Design review of the part built by this model. Coordinates are the model's own, in mm. Face numbers are marked on the shaded views. A direction names the side the tool comes from. Round coordinates to 2 decimals unless told otherwise and drop trailing zeros. Order: outer loops, then holes, each group sorted by start corner. A loop starts at its lowest first (then second) coordinate and runs counter-clockwise, first axis right, second up.
from build123d import *

# Parameters (mm, degrees)
F1_DEPTH = 25.4
F2_R     = 30.191545
F2_R_2   = 13.204956
F3_DEPTH = 46.73447
F4_W     = 33.58691
F4_H     = 33.58691
F5_DEPTH = 38.1


with BuildPart() as f1:
    # F0 (on Right) → F1 (new body)
    with BuildSketch(Plane.YZ):
        with BuildLine():
            ThreePointArc((-64.193385, -51.494292), (-34.284922, -33.102834), (-22.581748, 0))
            ThreePointArc((-22.581748, 0), (-34.284922, 33.102834), (-64.193385, 51.494292))
            ThreePointArc((-64.193385, 51.494292), (-127.917436, 0), (-64.193385, -51.494292))
        make_face()
        with BuildLine():
            ThreePointArc((-64.193385, 51.494292), (-34.284922, 33.102834), (-22.581748, 0))
            ThreePointArc((-22.581748, 0), (-34.284922, -33.102834), (-64.193385, -51.494292))
            Line((-64.193385, -51.494292), (59.976784, -24.834034))
            ThreePointArc((59.976784, -24.834034), (29.244732, 0), (59.976784, 24.834034))
            Line((59.976784, 24.834034), (-64.193385, 51.494292))
        make_face()
        with BuildLine():
            ThreePointArc((80.044732, 0), (74.400669, 15.964427), (59.976784, 24.834034))
            ThreePointArc((59.976784, 24.834034), (29.244732, 0), (59.976784, -24.834034))
            ThreePointArc((59.976784, -24.834034), (74.400669, -15.964427), (80.044732, 0))
        make_face()
    extrude(amount=F1_DEPTH)

    # F2 (on Right) → F3 (cut)
    with BuildSketch(Plane.YZ):
        with Locations((-75.075522, 0)):
            Circle(F2_R)
        with Locations((54.037802, 0)):
            Circle(F2_R_2)
    extrude(amount=F3_DEPTH, mode=Mode.SUBTRACT)

    # F4 (on Right) → F5 (join)
    with BuildSketch(Plane.YZ):
        with Locations((0.87742, -1.43759)):
            Rectangle(F4_W, F4_H)
    extrude(amount=F5_DEPTH)


solid = f1.part
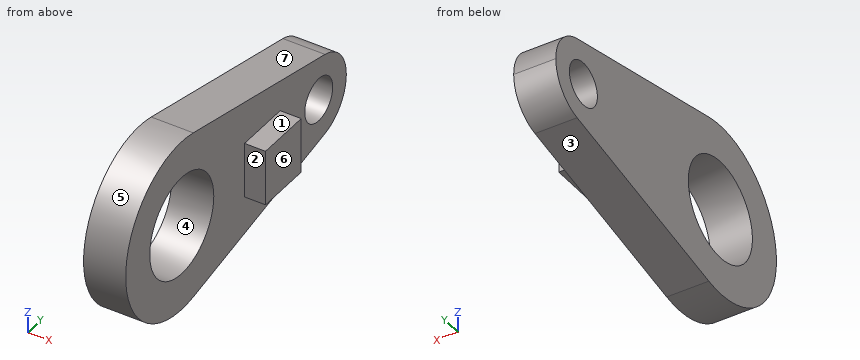
1) Take a section at B-B on y = 55. Give the boundary of the cut face in (x, z).
Results:
outline: (0, -25.9) - (25.4, -25.9) - (25.4, -13.17) - (0, -13.17) - close; (0, 13.17) - (25.4, 13.17) - (25.4, 25.9) - (0, 25.9) - close
2) For the marked faces 1, 2 and 3, list the 3-axis set-ups (+Z, -Z, +X, -X, +Y, -Y) from which the entire face can be reached by the end or side of a thin tool; tool diameter is ignored.
Results:
face 1: +Z, +X, +Y, -Y
face 2: +Z, -Z, +X, -Y
face 3: -Z, +X, -X, +Y
3) The part is to be moulded in two halves that separate along Z. For the marked faces 4, 5, 6 and 7, say which applies: released by +Z, released by -Z, zero draft, split by the parting line, or undercut.
Results:
face 4: undercut
face 5: split by the parting line
face 6: zero draft
face 7: released by +Z
4) Clearance check with flat-ended pins moving along their axes: P1, Ø4, axis at y = -11.5, z = -27.5, coming from the +X side; P2, Ø8, axis at x = 20.5, y = -27, coming from the +Z side; P3, Ø10, axis at x = 30.5, y = 3.5, coming from the -Z side. State where each tip first meets the part, or that it passes through.
Results:
P1: stops at x = 25.4
P2: stops at z = 44.37
P3: stops at z = -18.23
5) To check wall thickness, follow line 1 along Y through (x, z) = (9.5, 0); line 2 along X through (y, z) = (53, 17); line 3 along Y through (x, z) = (36, 6.5). State the ranges of each line that lie inside material, in increasing order.
Results:
line 1: y = -127.92 to -105.27, -44.88 to 40.83, 67.24 to 80.04
line 2: x = 0 to 25.4
line 3: y = -15.92 to 17.67
6) Take a section at C-C on z = -22.5. Give the boundary of the cut face in (x, y).
Results:
outline: (0, -122.87) - (25.4, -122.87) - (25.4, -95.21) - (0, -95.21) - close; (0, -54.94) - (25.4, -54.94) - (25.4, 66.43) - (0, 66.43) - close
7) Take a section at D-D on z = -33.5. Give the boundary of the cut face in (x, y).
Results:
outline: (0, -115.89) - (25.4, -115.89) - (25.4, 19.62) - (0, 19.62) - close
8) Take a section at A-A on x = 23. Give the boundary of the cut face in (y, z).
Results:
outline: (-64.19, -51.49) - (59.98, -24.83) arc R25.4 ccw to (80.04, 0) arc R25.4 ccw to (59.98, 24.83) - (-64.19, 51.49) arc R52.67 ccw (long way) to start; hole circle Ø60.38 at (-75.08, 0); hole circle Ø26.41 at (54.04, 0)
